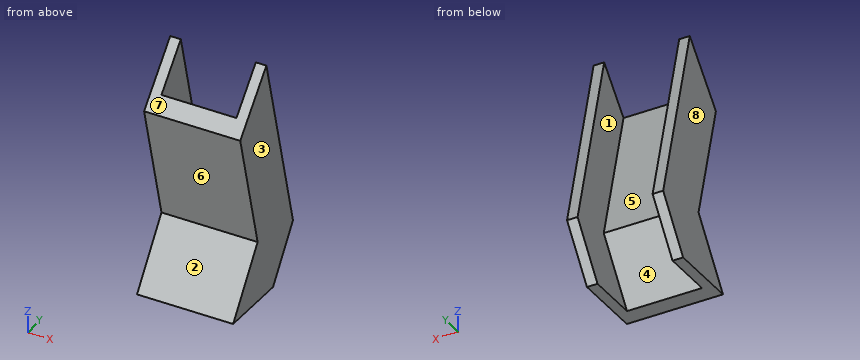
from build123d import *


with BuildPart() as part:
    # Sweep1: sweep along a path in Sketch2
    with BuildLine(Plane(origin=(0, 0, 0), x_dir=(0, 0, -1), z_dir=(1, 0, 0))) as sweep1_path:
        Line((0, 0), (-32.104520915, 22.431507437))
        Line((-32.104520915, 22.431507437), (-95.645680379, 6.47418981))
    # Sketch1 → Sweep1 (sweep)
    with BuildSketch(Plane.XY):
        Polygon((0, 0), (0, 36.574241376), (5.586518969, 36.574241376), (5.586518969, 9.514540119), (45.215887907, 9.514540119), (45.215887907, 36.574241376), (50.802406876, 36.574241376), (50.802406876, 0), align=None)
    sweep(path=sweep1_path.line, transition=Transition.RIGHT)


solid = part.part
The model under review builds one solid part; all positions refer to its coordinate system, in mm. Face numbers are marked on the shaded views. A direction names the side the tool comes from. Round coordinates to 2 decimals unless told otherwise and drop trailing zeros. Loops run counter-clockwise (first coordinate to the right, second up) from the corner with the lowest first, then second, coordinate; pieces in that order, holes last. Notation, with made-up numbers: (79, 72.25) -> (126, 72.25) arc R17 cw to (126, 78.25) -> close; hole circle Ø6 at (0, 59). An arc over 180 degrees is marked (long way). Return JSON: item names as keys, results as strings.
(1) For pin 1 (6 mm diameter, centred on x = 22, y = 9, fed in from +Z); pin 2 (1.5 mm diameter, centred on x = 30, z = 28, fed in from +Y); pin 3 (4 mm diameter, centred on x = 40.5, y = 14, fed in from -Z), all flat-tipped, find the tip position at first contact; note any pin that passes through.
Solved:
{"pin 1": "z = 102.01", "pin 2": "y = 29.6", "pin 3": "z = 3.56"}
(2) Add section A-A on y = 46. Write out the cut boundary in (x, z), plus the area to 3 significant figures.
Solved:
{"outline": "(0, 13.49) -> (5.59, 13.49) -> (5.59, 61.35) -> (0, 61.35) -> close; (45.22, 13.49) -> (50.8, 13.49) -> (50.8, 61.35) -> (45.22, 61.35) -> close", "area": "535 mm2"}
(3) Add section C-C on z = 97.5. Write out the cut boundary in (x, y), plus the area to 3 significant figures.
Solved:
{"outline": "(0, 8.08) -> (50.8, 8.08) -> (50.8, 36.92) -> (45.22, 36.92) -> (45.22, 14.05) -> (5.59, 14.05) -> (5.59, 36.92) -> (0, 36.92) -> close", "area": "559 mm2"}
(4) For line 1 (X direction, y = 33.5, z = 77.5); line 2 (Y direction, x = 10, z = 33.5); line 3 (Y direction, x = 2.5, z = 21), list the stretches that pass through material, from the lowest coordinate up.
Solved:
{"line 1": "0 to 5.59, 45.22 to 50.8", "line 2": "22.08 to 30.12", "line 3": "14.67 to 51.25"}
(5) Add section B-B on x = 41. Write out the cut boundary in (y, z).
Solved:
{"outline": "(0, 0) -> (9.51, 0) -> (30.86, 30.55) -> (12.71, 102.83) -> (6.47, 95.65) -> (22.43, 32.1) -> close"}
(6) Add section D-D on y = 38. Write out the cut boundary in (x, z).
Solved:
{"outline": "(0, 2.04) -> (5.59, 2.04) -> (5.59, 93.2) -> (0, 93.2) -> close; (45.22, 2.04) -> (50.8, 2.04) -> (50.8, 93.2) -> (45.22, 93.2) -> close"}
(7) The part is to be moulded in two halves that separate along X. For the marked faces 1, 2 and 3, say which applies: released by +X, released by -X, zero draft, split by the parting line, or undercut.
Solved:
{"face 1": "undercut", "face 2": "zero draft", "face 3": "released by +X"}
(8) For the marked faces 4, 5, 6, 7 and 8, list the 3-axis set-ups (+Z, -Z, +X, -X, +Y, -Y) from which the entire face can be reached by the end or side of a thin tool; tool diameter is ignored.
Solved:
{"face 4": "-Z, +Y", "face 5": "+Z, +Y", "face 6": "+X, -X, -Y", "face 7": "+Z, +X, -X, -Y", "face 8": "+Z, -Z, -X, +Y, -Y"}
